```python
from build123d import *

# Parameters (mm, degrees)
SKETCH1_W          = 100
SKETCH1_H          = 22.1615
BASE_FLANGE1_DEPTH = 1.524
HEM1_START         = -50
HEM1_DEPTH         = 100
HEM1_2_DEPTH       = 100
CUT_EXTRUDE1_START = -52.42823759
SKETCH8_W          = 14
SKETCH8_H          = 6.223
CUT_EXTRUDE1_DEPTH = 94.856475179
LPATTERN1_COUNT    = 11
LPATTERN1_PITCH    = 28
CHAMFER1_SIZE      = 0.5
SKETCH9_R          = 1.8288
CUT_EXTRUDE2_DEPTH = 10
LPATTERN2_COUNT    = 6
LPATTERN2_PITCH    = 50.8
CHAMFER2_SIZE      = 1


# Read off the part's stored shape, not the designer's step: Hem1
# Sheet-metal steps are written as plain solids
with BuildPart() as part:
    # Sketch1 → Base-Flange1 (new body)
    with BuildSketch(Plane(origin=(0, 0, 0), x_dir=(1, 0, 0), z_dir=(0, 1, 0))):
        Rectangle(SKETCH1_W, SKETCH1_H)
    extrude(amount=-BASE_FLANGE1_DEPTH)

    # Hem1 outline → Hem1 (cut)
    with BuildSketch(Plane.YZ.offset(HEM1_START)):
        with BuildLine():
            Line((0, -11.08075), (0, -10.645306054))
            ThreePointArc((0, -10.645306054), (-1.116287945, -9.509043168), (-1.524, -7.96925))
            Line((-1.524, -7.96925), (-1.524, -11.08075))
            Line((-1.524, -11.08075), (0, -11.08075))
        make_face()
    extrude(amount=HEM1_DEPTH, mode=Mode.SUBTRACT)

    # Hem1 2 outline → Hem1 2 (add)
    with BuildSketch(Plane.YZ.offset(HEM1_START)):
        with BuildLine():
            Line((0.272523279, -5.149273321), (0.916593509, -6.530486388))
            ThreePointArc((0.916593509, -6.530486388), (2.92638392, -8.822213128), (0, -7.96925))
            Line((0, -7.96925), (0, -10.645306054))
            ThreePointArc((0, -10.645306054), (4.69518189, -8.123345818), (0.272523279, -5.149273321))
        make_face()
    extrude(amount=HEM1_2_DEPTH)

    # Sketch8 → Cut-Extrude1 (cut)
    with BuildSketch(Plane(origin=(0, 0, 0), x_dir=(1, 0, 0), z_dir=(0, 1, 0)).offset(CUT_EXTRUDE1_START)):
        with Locations((-43, 7.96925)):
            Rectangle(SKETCH8_W, SKETCH8_H)
    cut_extrude1 = extrude(amount=CUT_EXTRUDE1_DEPTH, mode=Mode.SUBTRACT)

    # LPattern1: Cut-Extrude1 ×11
    with Locations(*[(i * LPATTERN1_PITCH, 0, 0) for i in range(1, LPATTERN1_COUNT)]):
        add(cut_extrude1, mode=Mode.SUBTRACT)

    # Chamfer1
    chamfer1_edges = [part.edges().sort_by_distance(p)[0] for p in [
        (50, 2.92638392, -8.822213128),
        (-50, 0, 3.1115),
        (0, 0, 11.08075),
        (50, 0, 1.55575),
    ]]
    chamfer(chamfer1_edges, length=CHAMFER1_SIZE)

    # Sketch9 → Cut-Extrude2 (cut)
    with BuildSketch(Plane(origin=(0, 0, 0), x_dir=(1, 0, 0), z_dir=(0, 1, 0))):
        with Locations(Location((-24.6, -3.14325, 0), (0, 0, 270))):
            Circle(SKETCH9_R)
    cut_extrude2 = extrude(amount=-CUT_EXTRUDE2_DEPTH, mode=Mode.SUBTRACT)

    # LPattern2: Cut-Extrude2 ×6
    with Locations(*[(i * LPATTERN2_PITCH, 0, 0) for i in range(1, LPATTERN2_COUNT)]):
        add(cut_extrude2, mode=Mode.SUBTRACT)

    # Chamfer2
    chamfer2_edges = [part.edges().sort_by_distance(p)[0] for p in [
        (-24.6, 0, 1.31445),
        (26.2, 0, 1.31445),
    ]]
    chamfer(chamfer2_edges, length=CHAMFER2_SIZE)


solid = part.part
```
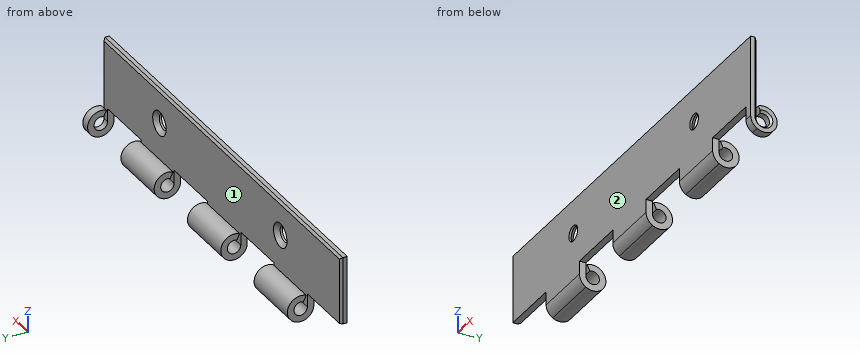
The listing builds one solid part. Answer for the finished solid, in the listing's coordinates (mm). Face numbers are marked on the shaded views. A direction names the side the tool comes from. Coordinates: 2 decimals unless noted, no trailing zeros. Loops run counter-clockwise (first coordinate to the right, second up) from the corner with the lowest first, then second, coordinate; pieces in that order, holes last. Notation, with made-up numbers: (13.25, 26) -> (24.25, 26) arc R28 ccw to (24.25, 57) -> close; hole circle Ø6 at (27.5, 38.5). An arc over 180 degrees is marked (long way). Use one line per item in the form item = value. Start each with the question number.
Item 1: The part is cut by section C-C on z = -1.5. Determine the outline of the cut face in (x, y), then the cut area to 3 significant figures.
Item 2: The part is cut by section B-B on x = -4. Determine the outline of the cut face in (y, z) (1 decimal).
Item 3: Flat-ended cylindrical pins translate along their axes: pin 1 Ø3 at (y, z) = (1.59, -7.97) entering from -X; pin 2 Ø1.7 at (x, y) = (-15, -0.5) entering from -Z; pin 3 Ø3 at (y, z) = (2.5, -6.5) entering from -X; pin 4 Ø1 at (x, z) = (14, 0) entering from +Y. Find the tip coordinate at first contact, or state that the pin passes through.
Item 4: A tool of negligible diameter and unlimited length cuts with its end or side. For the marked faces 1 and 2, from which of +Z, -Z, +X, -X, +Y, -Y can it reach the whole face along a straight path? Write none if from no direction.
Item 5: The part is cut by section A-A on x = -24.6. Determine the outline of the cut face in (y, z) (1 decimal), then the cut area to 3 significant figures.
Item 6: The part is cut by section D-D on x = 39.5. Determine the outline of the cut face in (y, z).
Item 7: Consider L1, parallel to X at y = 0.25, z = -9.75; L2, parallel to Z at x = -5, y = 1.5; L3, parallel to X at y = 3.5, z = -7.75. Determine where each line is inside the solid, lowest interval first. Write a range as [from, to].
Answer key:
q1.outline = (-50, -1.52) -> (50, -1.52) -> (50, -0.5) -> (49.5, 0) -> (-49.5, 0) -> (-50, -0.5) -> close
q1.area = 152 mm2
q2.outline = (-1.5, -8) arc R3.1 ccw (long way) to (0.3, -5.1) -> (0.9, -6.5) arc R1.6 cw (long way) to (0, -8) -> (0, 10.6) -> (-0.5, 11.1) -> (-1.5, 11.1) -> close
q3.pin_1 = through
q3.pin_2 = -4.86
q3.pin_3 = -36
q3.pin_4 = 0
q4.face_1 = +Z, +X, -X
q4.face_2 = +Z, -Z, +X, -X, -Y
q5.outline = (-1.5, -8) arc R3.1 ccw (long way) to (0.3, -5.1) -> (0.9, -6.5) arc R1.6 cw (long way) to (0, -8) -> (0, 0.3) -> (-1, 1.3) -> (-1.5, 1.3) -> close; (-1.5, 5) -> (-1, 5) -> (0, 6) -> (0, 10.6) -> (-0.5, 11.1) -> (-1.5, 11.1) -> close
q5.area = 40.8 mm2
q6.outline = (-1.52, -4.86) -> (0, -4.86) -> (0, 10.58) -> (-0.5, 11.08) -> (-1.52, 11.08) -> close
q7.L1 = [-36, -22], [-8, 6], [20, 34], [48, 50]
q7.L2 = [-11.08, -9.55], [-6.38, -4.86]
q7.L3 = [-36, -22], [-8, 6], [20, 34], [48, 49.84]
